Model file for the job. Use its own axes, mm. Coordinates: 2 decimals unless noted, no trailing zeros. Order: outer loops, then holes, each group sorted by start corner. A loop starts at its lowest first (then second) coordinate and runs counter-clockwise, first axis right, second up. Notation, with made-up numbers: (4.5, 30.25) -> (18.5, 30.25) arc R18 ccw to (18.5, 59.25) -> close; hole circle Ø5 at (-5.75, 78). An arc over 180 degrees is marked (long way). Return JSON: item names as keys, results as strings. Group by question number.
1) Pull direction Z, two halves, no side cores. Call faces 1 (the cylindrical face through (0, 2, 3)), 2 (the flat face through (-1, 4, -42)), 3 (the cylindrical face through (-1.05, 1.97, -0.33)): +Z half, -Z half, draft (parallel to the pull), parting line (faces both ways), or undercut.
2) Cut at C-C (z = -65.5). Write the cut outline in (x, y).
3) Flat gauge pin, fed straight in: pin 1 (2 mm diameter, centred on x = 1.5, y = 3.5, fed in from -Z). Where does the tip first touch, or does it go through?
4) Cut at B-B (y = 1.4). Write the cut outline in (x, z).
5) Cut at A-A (x = 2). Write the cut outline in (y, z), and give its area (3 significant figures).
6) Probe line 1 (X direction, y = 2.3, z = -85.9); line 2 (Z direction, x = -1, y = 3.55); line 3 (X direction, y = 2.45, z = -34). List the from-to ranges inside material, lowest first.
Autodesk Inventor part; units mm, degrees
ref_plane "YZ Plane" through (0, 0, 0) normal (1, 0, 0) x (0, 1, 0)
ref_plane "XZ Plane" through (0, 0, 0) normal (0, 1, 0) x (-1, 0, 0)
ref_plane "XY Plane" through (0, 0, 0) normal (0, 0, 1) x (1, 0, 0)
sketch "Sketch1" plane through (0, 0, 0) normal (0, 1, 0) x (-1, 0, 0)
  line L0 (0, 0) -> (0, -85.9) construction
  line L1 (3, 0) -> (3, -85.9)
  line L2 (-3, -85.9) -> (-3, 0)
  arc A0 (3, 0) -> (-3, 0) centre (0, 0) ccw
  arc A1 (-3, -85.9) -> (3, -85.9) centre (0, -85.9) ccw
  circle A2 centre (0, 0) radius 1.1
  circle A3 centre (0, -85.9) radius 1.1
  arc A4 (-3, -85.9) -> (-3, 0) centre (-299.9096, -42.95) ccw
  arc A5 (3, -85.9) -> (3, 0) centre (-293.9096, -42.95) ccw
  point P0 (0, -42.95)
  dimension "d0" = 2.2
  dimension "d1" = 2.2
  dimension "d2" = 6
  dimension "d3" = 85.9
  dimension "d10" = 300
  dimension "d11" = 300
extrude "Extrusion1" add sketch "Sketch1" along normal blind 4 contours A5 L1 | L1 A1 A4 A0
Answers below:
{
 "1": {"face 1": "+Z half", "face 2": "draft", "face 3": "undercut"},
 "2": {"outline": "(-5.24, 0) -> (0.76, 0) -> (0.76, 4) -> (-5.24, 4) -> close"},
 "3": {"pin 1": "stops at z = -88.86"},
 "4": {"outline": "(-3, -85.9) arc R3 ccw to (3, -85.9) arc R300 cw to (3, 0) arc R3 ccw to (-3, 0) arc R300 ccw to start; hole circle Ø2.2 at (0, -85.9); hole circle Ø2.2 at (0, 0)"},
 "5": {"outline": "(0, -88.14) -> (4, -88.14) -> (4, -78.3) -> (0, -78.3) -> close; (0, -7.6) -> (4, -7.6) -> (4, 2.24) -> (0, 2.24) -> close", "area": "78.7 mm^2"},
 "6": {"line 1": "x = -3 to -1.1, 1.1 to 3", "line 2": "z = -88.73 to -86.36, -85.44 to -0.46, 0.46 to 2.83", "line 3": "x = -5.96 to 0.04"}
}
